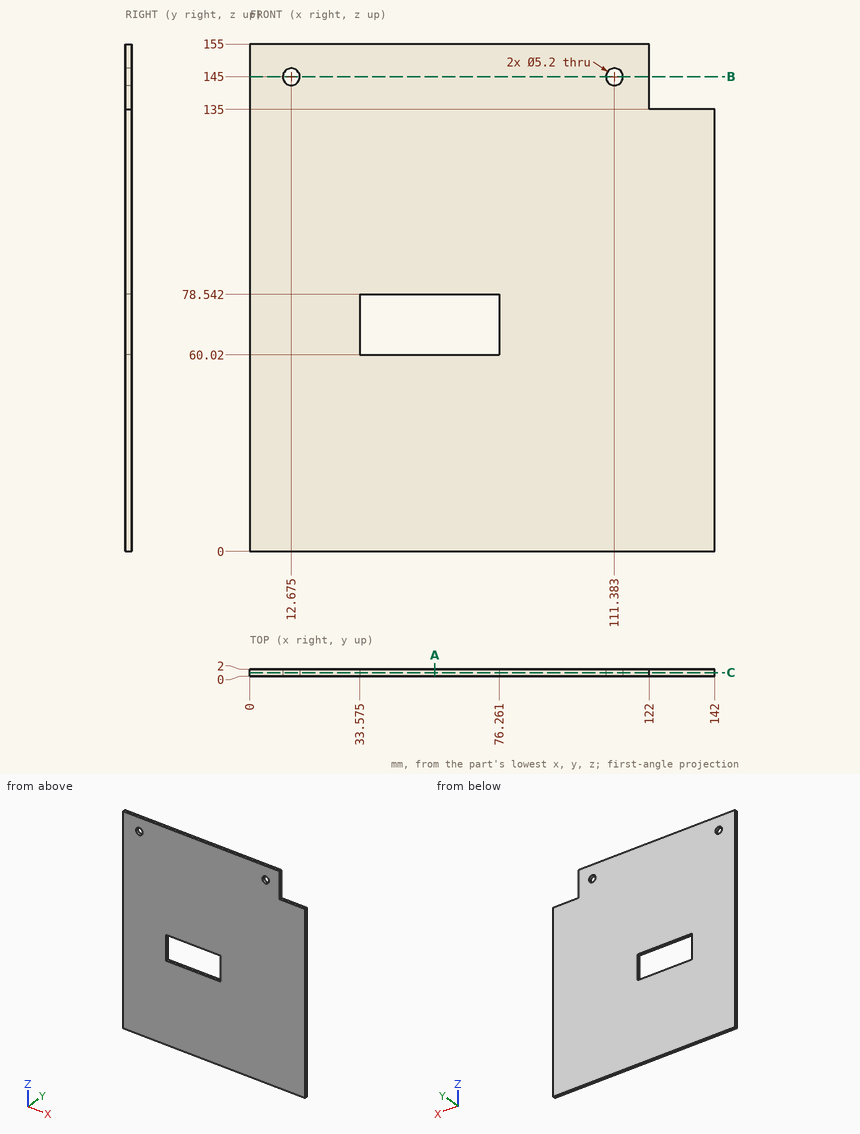
The figure shows three views and two pictorial views of one solid part (mm, origin at its lowest corner). Answer the questions. Round coordinates to 2 decimals unless told otherwise and drop trailing zeros. Order: outer loops, then holes, each group sorted by start corner. A loop starts at its lowest first (then second) coordinate and runs counter-clockwise, first axis right, second up. Notation, with made-up numbers: M 77.5,-35 L 87.5,-35 A16 cw 87.5,-31 Z; hole C -35,70.25 d11. An arc over 180 degrees is marked long. Put each result on its own line as item: value. Start each with the question number.
Q1. Section A-A, the plane x = 56.5 is taken. Write down the section's boundary in (y, z).
Q2. Straight lines are drawn through the part: L1, parallel to X at y = 0.75, z = 145 (1 decimal); L2, parallel to X at y = 1.85, z = 74 (1 decimal); L3, parallel to Z at x = 40.5, y = 0.6. For each, find the intervals that lie inside material, in ascending order. Write a range as [from, to].
Q3. Flat-ended cylindrical pins translate along their axes: pin 1 (4.5 mm diameter, centred on x = 111.38, z = 145, fed in from +Y); pin 2 (0.6 mm diameter, centred on y = 1, z = 149.5, fed in from +X). Find the tip coordinate at first contact, or state that the pin passes through.
Q4. Section C-C, the plane y = 1 is taken. Write down the section's boundary in (x, z) (1 decimal), and give its area (3 significant figures).
Q5. Section B-B, the plane z = 145 is taken. Write down the section's boundary in (x, y) (1 decimal).
Findings below:
1. outline: M 0,0 L 2,0 L 2,60.02 L 0,60.02 Z; M 0,78.54 L 2,78.54 L 2,155 L 0,155 Z
2. L1: x = [0, 10.1], [15.3, 108.8], [114, 122]
2. L2: x = [0, 33.6], [76.3, 142]
2. L3: z = [0, 60.02], [78.54, 155]
3. pin 1: passes through
3. pin 2: stops at x = 122
4. outline: M 0,0 L 142,0 L 142,135 L 122,135 L 122,155 L 0,155 Z; hole C 12.7,145 d5.2; hole M 33.6,60 L 76.3,60 L 76.3,78.5 L 33.6,78.5 Z; hole C 111.4,145 d5.2
4. area: 20,800 mm^2
5. outline: M 0,0 L 10.1,0 L 10.1,2 L 0,2 Z; M 15.3,0 L 108.8,0 L 108.8,2 L 15.3,2 Z; M 114,0 L 122,0 L 122,2 L 114,2 Z
